```python
from build123d import *

# Parameters (mm, degrees)
BOSS_EXTRUDE1_DEPTH = 1.5875
BOSS_EXTRUDE2_DEPTH = 101.6


with BuildPart() as part:
    # Sketch1 → Boss-Extrude1 (new, symmetric)
    with BuildSketch(Plane(origin=(0, 0, 0), x_dir=(1, 0, 0), z_dir=(0, 1, 0))):
        Polygon((-101.6, 0), (101.6, 0), (101.6, 76.2), (0, 76.2), align=None)
    extrude(amount=BOSS_EXTRUDE1_DEPTH, both=True)

    # Sketch2 → Boss-Extrude2 (add, symmetric)
    with BuildSketch(Plane(origin=(0, 0, 0), x_dir=(0, 0, -1), z_dir=(1, 0, 0))):
        with BuildLine():
            ThreePointArc((-0.007951018, -0.79375), (-0.017893832, -1.190684781), (-0.031813653, -1.5875))
            Line((-0.031813653, -1.5875), (0, -1.5875))
            Line((0, -1.5875), (-0.007951018, -0.79375))
        make_face()
        with BuildLine():
            Line((0, -1.5875), (0, 0))
            ThreePointArc((0, 0), (-0.001987804, -0.396894911), (-0.007951018, -0.79375))
            Line((-0.007951018, -0.79375), (0, -1.5875))
        make_face()
        with BuildLine():
            Line((0, 0), (0, 1.5875))
            Line((0, 1.5875), (-0.031813653, 1.5875))
            ThreePointArc((-0.031813653, 1.5875), (-0.007954212, 0.793909371), (0, 0))
        make_face()
    extrude(amount=BOSS_EXTRUDE2_DEPTH, both=True)


solid = part.part
```
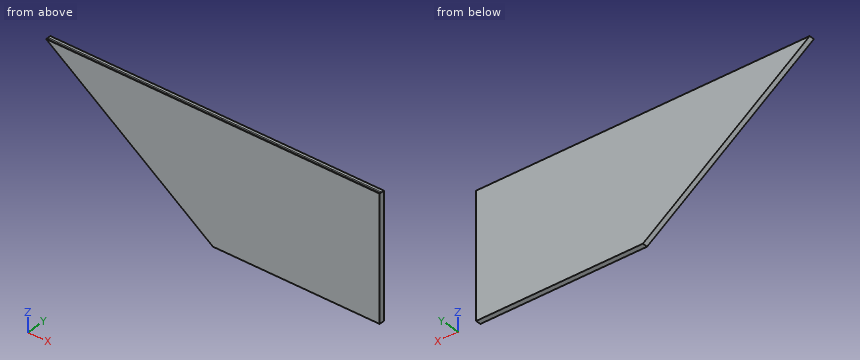
Source: CAD feature listing. Evaluate the final solid. Frame: model axes, mm. Round coordinates to 2 decimals unless told otherwise and drop trailing zeros. Order: outer loops, then holes, each group sorted by start corner. A loop starts at its lowest first (then second) coordinate and runs counter-clockwise, first axis right, second up. Notation, with made-up numbers: (-8.75, 28.25) -> (3.25, 28.25) arc R5 cw to (3.25, 37.25) -> close; hole circle Ø3 at (28.25, 21). An arc over 180 degrees is marked (long way). One line per item, written item: value. Start each with the question number.
Q1. Section query D-D (z = -28.5). Return the cut outline in (x, y).
Q2. Material intervals for probe 1 along Z at (x, y) = (84, 0.35); probe 2 along X at (y, z) = (-1.4, -25.5); probe 3 along Z at (x, y) = (-41, 1.1), sorted ascending.
Q3. Section query A-A (z = -64.5). Return the cut outline in (x, y).
Q4. Section query B-B (x = -5). Return the cut outline in (y, z).
Findings below:
1. outline: (-63.6, -1.59) -> (101.6, -1.59) -> (101.6, 1.59) -> (-63.6, 1.59) -> close
2. probe 1: -76.2 to 0
2. probe 2: -67.6 to 101.6
2. probe 3: -45.45 to 0.02
3. outline: (-15.6, -1.59) -> (101.6, -1.59) -> (101.6, 1.59) -> (-15.6, 1.59) -> close
4. outline: (-1.59, -72.45) -> (1.59, -72.45) -> (1.59, 0.03) arc R39.62 cw to (0, 0) arc R39.62 cw to (-0.79, 0.01) arc R39.62 cw to (-1.59, 0.03) -> close
